```python
from build123d import *

# Parameters (mm, degrees)
SKETCH_1_W             = 82
SKETCH_1_H             = 57
EXTRUDE_1_DEPTH        = 14
SKETCH_2_W             = 12.989846737
SKETCH_2_H             = 9.461740216
EXTRUDE_2_DEPTH        = 8.2
PATTERN_LINEAR_1_COUNT = 4
PATTERN_LINEAR_1_PITCH = 22


with BuildPart() as part:
    # 草图1 → 凸台-拉伸1 (new body)
    with BuildSketch(Plane(origin=(0, 0, 0), x_dir=(1, 0, 0), z_dir=(0, 1, 0))):
        Rectangle(SKETCH_1_W, SKETCH_1_H)
    extrude(amount=EXTRUDE_1_DEPTH)

    # 草图2 → 凸台-拉伸2 (add)
    with BuildSketch(Plane.XY.offset(28.5)):
        with Locations((-32.634985321, 2.629958968)):
            Rectangle(SKETCH_2_W, SKETCH_2_H)
    extrude_2 = extrude(amount=EXTRUDE_2_DEPTH)

    # 阵列(线性)1: 凸台-拉伸2 ×4
    with Locations(*[(i * PATTERN_LINEAR_1_PITCH, 0, 0) for i in range(1, PATTERN_LINEAR_1_COUNT)]):
        add(extrude_2)


solid = part.part
```
Geometry: final body of the model. Coordinates: model frame, mm. A direction names the side the tool comes from. Coordinates: 2 decimals unless noted, no trailing zeros. Order: outer loops, then holes, each group sorted by start corner. A loop starts at its lowest first (then second) coordinate and runs counter-clockwise, first axis right, second up. Notation, with made-up numbers: M -24,33.5 L 35,33.5 A10 cw 35,48.5 Z; hole C 66.25,-20 d11. An arc over 180 degrees is marked long. Answer in a Markdown table with one row per item. Add a question column.
Q1. Section query A-A on y = 4.5. Return the cut outline in (x, z), and give its area (3 significant figures).
Q2. Section query B-B on x = -16. Return the cut outline in (y, z).
Q3. Section query D-D on y = 12.5. Return the cut outline in (x, z), and give its area (3 significant figures).
Q4. Contact query for flat-ended pins moving along their axis: P1, Ø1.1, axis at x = -11, y = -1.5, coming from the -Z side; P2, Ø2.5, axis at y = 3.5, z = 32, coming from the -X side; P3, Ø6.5, axis at x = 9, z = 33, coming from the +Y side. Output: stop coordinate, or through.
Q5. Line query: L1, parallel to Y at x = -24.5, z = -16; L2, parallel to Z at x = -7, y = 9.5; L3, parallel to Y at x = 8, z = 30.5. Output: solid intervals per line, ascending.
Q6. Mould query, pull axis X, two halves, no side actions, for faces 1 (the flat face through (4.87, 3, 33)), 2 (the flat face through (39.86, 3, 33)), 3 (the flat face through (-11, -2.101, 33)), 4 (the flat face through (-17.13, 3, 33)). Classes: released by +X, released by -X, zero draft, split by the parting line, or undercut.
Q7. Section query C-C on z = -11. Return the cut outline in (x, y), and give its area (3 significant figures).
Q8. Reachability of faces 5 (the flat face through (-39.13, 3, 33)), 6 (the flat face through (26.87, 3, 33)), 7 (the flat face through (33, 7.361, 33)), 8 (the flat face through (-11, -1, 28.5)) from +Z, -Z, +X, -X, +Y, -Y: full face, straight path, thin tool, end or side. Return the list, or none.
Completed:
| question | item | result |
|---|---|---|
| 1 | outline | M -41,-28.5 L 41,-28.5 L 41,28.5 L 39.86,28.5 L 39.86,36.7 L 26.87,36.7 L 26.87,28.5 L 17.86,28.5 L 17.86,36.7 L 4.87,36.7 L 4.87,28.5 L -4.14,28.5 L -4.14,36.7 L -17.13,36.7 L -17.13,28.5 L -26.14,28.5 L -26.14,36.7 L -39.13,36.7 L -39.13,28.5 L -41,28.5 Z |
| 1 | area | 5,100 mm2 |
| 2 | outline | M -2.1,28.5 L 0,28.5 L 0,-28.5 L 14,-28.5 L 14,28.5 L 7.36,28.5 L 7.36,36.7 L -2.1,36.7 Z |
| 3 | outline | M -41,-28.5 L 41,-28.5 L 41,28.5 L -41,28.5 Z |
| 3 | area | 4,670 mm2 |
| 4 | P1 | stops at z = 28.5 |
| 4 | P2 | stops at x = -39.13 |
| 4 | P3 | stops at y = 7.36 |
| 5 | L1 | y = 0 to 14 |
| 5 | L2 | z = -28.5 to 28.5 |
| 5 | L3 | y = -2.1 to 7.36 |
| 6 | face 1 | undercut |
| 6 | face 2 | released by +X |
| 6 | face 3 | zero draft |
| 6 | face 4 | undercut |
| 7 | outline | M -41,0 L 41,0 L 41,14 L -41,14 Z |
| 7 | area | 1,150 mm2 |
| 8 | face 5 | +Z, -X, +Y, -Y |
| 8 | face 6 | +Z, +Y, -Y |
| 8 | face 7 | +Z, +X, -X, +Y |
| 8 | face 8 | -Z, +X, -X, -Y |
